Check sheet for the modelled part. Datum: model origin and axes. Units: mm. Face numbers are marked on the shaded views. A direction names the side the tool comes from. Give positions to 0.01 mm unless a question says otherwise; leave off trailing zeros. Write each loop counter-clockwise with the first axis right and the second up, starting at its lowest first coordinate (ties: lowest second). Pieces come first, ordered by that corner, then holes. Notation, with made-up numbers: M 55,72.25 L 59,72.25 A20 cw 59,89.25 Z; hole C 38,13 d8. An arc over 180 degrees is marked long. Write item = value, one per line. Start each with the question number.
1) Cross-section at A-A, the plane x = -9.5. Record the cut outline in (y, z).
2) Cross-section at B-B, the plane y = 5.75. Record the cut outline in (x, z), plus the area to 3 significant figures.
3) Go/stop test with flat-tipped pins: pin 1 (8.5 mm diameter, centred on x = -1.5, y = 9, fed in from +Z); pin 2 (3 mm diameter, centred on x = 8, y = 6, fed in from +Z); pin 3 (5 mm diameter, centred on x = 4, y = 17.5, fed in from -Z); pin 4 (8 mm diameter, centred on y = 10, z = 14.5, fed in from +X). Record where each tip stops, or that it passes through.
4) Cross-section at C-C, the plane x = 7.25. Record the cut outline in (y, z), plus the area to 3 significant figures.
5) Scan lines: line 1 along Z through (x, y) = (0.5, 4.5); line 2 along X through (y, z) = (10.75, 1); line 3 along Y through (x, z) = (8.5, 11.75). Record each from-to range of solid material in increasing order. Write a range as [from, to].
6) Access from +Z, -Z, +X, -X, +Y, -Y to the whole of each face (thin tool, end or side, straight path). Record for the marked faces 1 and 2.
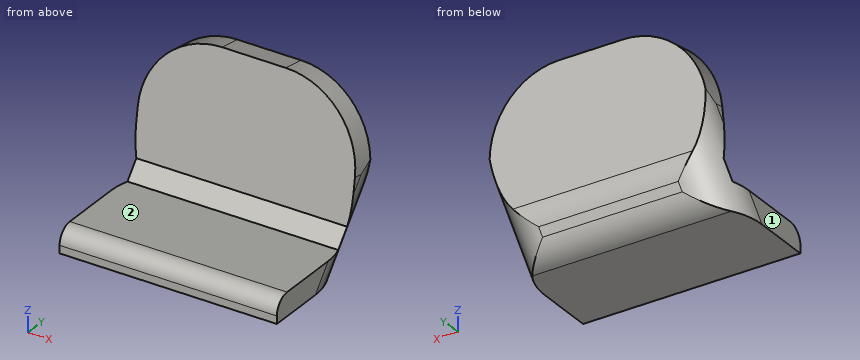
```python
from build123d import *

# Parameters (mm, degrees)
F0_W        = 28
F0_H        = 3
F3_R        = 9.8982756057
F4_R        = 2
F5_T1_DEPTH = 29.9393718709
F5_T3_DEPTH = 39.6309025582
F5_T5_DEPTH = 35.0165294795


# Not quite as in the source:
# - a fillet or chamfer that OpenCascade refuses, or shapes differently, is made with other operations: its cross-section is extruded or revolved along the edge and cut away or added


with BuildPart() as f2:
    # F2: sweep along a path in F1
    with BuildLine(Plane.YZ) as f2_path:
        Line((0, 0), (13.3813479915, 0))
        Line((13.3813479915, 0), (15.8422850072, 2.9223633464))
        Line((15.8422850072, 2.9223633464), (18.3032229543, 18.9184583724))
    # F0 (on Front) → F2 (sweep)
    with BuildSketch(Plane.XZ):
        Rectangle(F0_W, F0_H)
    sweep(path=f2_path.line, transition=Transition.RIGHT)

    # F3
    f3_edges = [f2.edges().sort_by_distance(p)[0] for p in [
        (14, 18.303223, 18.918458),
        (-14, 18.303223, 18.918458),
    ]]
    fillet(f3_edges, radius=F3_R)

    # F4
    f4_edges = [f2.edges().sort_by_distance(p)[0] for p in [
        (0, 0, 1.5),
    ]]
    fillet(f4_edges, radius=F4_R)

    # F5: fillet of radius 5 on 4 edges, made by hand

    # F5_s2 → F5_t1 (cut)
    with BuildSketch(Plane(origin=(0, -2.9491433719, -3.5021085214), x_dir=(1, 0, 0), z_dir=(0, 0.6441356632, 0.7649112677))):
        with BuildLine():
            ThreePointArc((-9, 11.7355438551), (-12.5355339059, 10.271077761), (-14, 6.7355438551))
            Line((-14, 6.7355438551), (-14, 11.7355438551))
            Line((-14, 11.7355438551), (-9, 11.7355438551))
        make_face()
        with BuildLine():
            ThreePointArc((14, 6.7355438551), (12.5355339059, 10.271077761), (9, 11.7355438551))
            Line((9, 11.7355438551), (14, 11.7355438551))
            Line((14, 11.7355438551), (14, 6.7355438551))
        make_face()
    extrude(amount=F5_T1_DEPTH, mode=Mode.SUBTRACT)

    # F5_s4 → F5_t3 (cut)
    with BuildSketch(Plane.YZ.offset(-19.8154512791)):
        with BuildLine():
            ThreePointArc((11.7530216334, -1.5), (13.8621219652, -1.0333978195), (15.5775779716, 0.279321684))
            Line((15.5775779716, 0.279321684), (14.079202145, -1.5))
            Line((14.079202145, -1.5), (11.7530216334, -1.5))
        make_face()
    extrude(amount=F5_T3_DEPTH, mode=Mode.SUBTRACT)

    # F5_s6 → F5_t5 (cut)
    with BuildSketch(Plane.YZ.offset(-17.5082647397)):
        with BuildLine():
            ThreePointArc((16.356908347, 1.2047767074), (17.0849215873, 2.3580628903), (17.4742104853, 3.6651690265))
            Line((17.4742104853, 3.6651690265), (17.2608277209, 2.2781811991))
            Line((17.2608277209, 2.2781811991), (16.356908347, 1.2047767074))
        make_face()
    extrude(amount=F5_T5_DEPTH, mode=Mode.SUBTRACT)


solid = f2.part
```
Reply:
q1.outline = M 0,-1.5 L 11.75,-1.5 A5 ccw 15.24,-0.09 L 16.66,1.6 A5 ccw 17.47,3.67 L 19.54,17.11 L 16.58,17.56 L 14.42,3.57 L 12.68,1.5 L 2,1.5 A2 ccw 0,-0.5 Z
q2.outline = M -14,-1.5 L 14,-1.5 L 14,1.5 L -14,1.5 Z
q2.area = 84.0 mm2
q3.pin_1 = 2.17
q3.pin_2 = 1.5
q3.pin_3 = -0.3
q3.pin_4 = through
q4.outline = M 0,-1.5 L 11.75,-1.5 A5 ccw 15.58,0.28 L 16.36,1.2 A5 ccw 17.47,3.67 L 19.71,18.18 L 16.74,18.64 L 14.42,3.57 L 12.68,1.5 L 2,1.5 A2 ccw 0,-0.5 Z
q4.area = 96.8 mm2
q5.line_1 = [-1.5, 1.5]
q5.line_2 = [-13.93, 13.93]
q5.line_3 = [15.68, 18.72]
q6.face_1 = +Z, -Z, -X, +Y, -Y
q6.face_2 = +Z, +X, -X, -Y
